Input: part model. Units: mm. Frame: model coordinates. A direction names the side the tool comes from. Coordinates: 2 decimals unless noted, no trailing zeros. Order: outer loops, then holes, each group sorted by start corner. A loop starts at its lowest first (then second) coordinate and runs counter-clockwise, first axis right, second up. Notation, with made-up numbers: (66, 3) - (122, 3) arc R32 cw to (122, 36) - close; hole circle Ø3 at (65, 4). An arc over 180 degrees is marked (long way). One line per question, with ' | ' between items. Start each with the question number.
Autodesk Fusion 360 part; units mm, degrees
sketch "Skizze1" plane through (0, 0, 0) normal (0, 1, 0) x (1, 0, 0)
  line L0 (25, 16) -> (-25, 16)
  line L1 (-25, 16) -> (-25, -16)
  line L2 (-25, -16) -> (25, -16)
  line L3 (25, -16) -> (25, 16)
  line L4 (25, 16) -> (-25, -16) construction
  line L5 (-25, 16) -> (25, -16) construction
  dimension "d1" = 50
  dimension "d2" = 32
extrude "Extrusion1" add sketch "Skizze1" along normal blind 1
sketch "Skizze2" plane through (0, 1, 0) normal (0, 1, 0) x (-1, 0, 0)
  line L0 (-25, 16) -> (-25, -16)
  line L1 (-25, -16) -> (25, -16)
  line L2 (25, -16) -> (25, 16)
  line L3 (25, 16) -> (-25, 16)
  circle A0 centre (0, 0) radius 4.9
  line L4 (0, 0) -> (0, -16) construction
  line L5 (0, 0) -> (-14.6371, -14.6371) construction
  line L6 (0, 0) -> (-14.6371, 14.6371) construction
  arc A1 (-7.0711, 7.0711) -> (-9.051, 9.051) centre (-8.061, 8.061) ccw
  arc A2 (-12.6572, 12.6572) -> (-14.6371, 14.6371) centre (-13.6472, 13.6472) ccw
  arc A3 (-9.051, 9.051) -> (-9.051, -9.051) centre (0, 0) ccw
  arc A4 (-7.0711, 7.0711) -> (-7.0711, -7.0711) centre (0, 0) ccw
  arc A5 (-14.6371, -14.6371) -> (-12.6572, -12.6572) centre (-13.6472, -13.6472) ccw
  arc A6 (-9.051, -9.051) -> (-7.0711, -7.0711) centre (-8.061, -8.061) ccw
  arc A7 (-12.6572, 12.6572) -> (-12.6572, -12.6572) centre (0, 0) ccw
  arc A8 (-14.6371, 14.6371) -> (-14.6371, -14.6371) centre (0, 0) ccw
  arc A9 (12.6572, -12.6572) -> (12.6572, 12.6572) centre (0, 0) ccw
  arc A10 (14.6371, -14.6371) -> (14.6371, 14.6371) centre (0, 0) ccw
  line L7 (25, 16) -> (25, -16)
  line L8 (0, 0) -> (14.6371, 14.6371) construction
  line L9 (25, -16) -> (-25, -16)
  arc A11 (9.051, -9.051) -> (9.051, 9.051) centre (0, 0) ccw
  arc A12 (12.6572, -12.6572) -> (14.6371, -14.6371) centre (13.6472, -13.6472) ccw
  arc A13 (7.0711, -7.0711) -> (7.0711, 7.0711) centre (0, 0) ccw
  line L10 (0, 0) -> (14.6371, -14.6371) construction
  arc A14 (9.051, 9.051) -> (7.0711, 7.0711) centre (8.061, 8.061) ccw
  line L11 (-25, 16) -> (25, 16)
  arc A15 (7.0711, -7.0711) -> (9.051, -9.051) centre (8.061, -8.061) ccw
  arc A16 (14.6371, 14.6371) -> (12.6572, 12.6572) centre (13.6472, 13.6472) ccw
  dimension "d6" = 9.8
  dimension "d7" = 2.8
  dimension "d8" = 5.1
  dimension "d9" = 5.1
  dimension "d10" = 2.8
  dimension "d11" = 45
extrude "Extrusion2" add sketch "Skizze2" along normal blind 1 contours A0 | A1 A3 A4 A6 | A2 A5 A7 A8 | A9 A10 A12 A16 | A11 A13 A14 A15
equation "d9 = d8"
equation "d10 = d7"
(1) Section A-A (y = 1.35). Output: boundary loops of the cut face in (x, z), then the cut area to 3 significant figures.
(2) Material intervals for line 1 along X through (y, z) = (1.45, -5); line 2 along X through (y, z) = (1.95, 2.5); line 3 along X through (y, z) = (1.15, -2), sorted ascending. Write a range as from..to.
(3) Draft query along Z for faces 3 (the face through (12.68, 1.49, 14.66)), 4 (the face through (-12.64, 1.49, 14.62)), 5 (the face through (0, 2, 0)), 6 (the face through (-0.3, 0.5, 16)). Return one class per face: +Z half, -Z half, draft (parallel to the pull), parting line (faces both ways), or undercut.
(4) Reachability of faces 1 (the face through (7.05, 1.49, -9.03)), 2 (the face through (-10.4, 2, 0.1)) from +Z, -Z, +X, -X, +Y, -Y: full face, straight path, thin tool, end or side. Return the list, or none.
(5) Section C-C (z = 0). Output: boundary loops of the cut face in (x, y).
(6) Section D-D (x = -20). Output: boundary loops of the cut face in (y, z).
(7) Section B-B (x = 0). Output: boundary loops of the cut face in (y, z), then the cut area to 3 significant figures.
Worked answers:
1) outline: (-14.64, -14.64) arc R1.4 ccw to (-12.66, -12.66) arc R17.9 cw to (-12.66, 12.66) arc R1.4 ccw to (-14.64, 14.64) arc R20.7 ccw to start; (-9.05, -9.05) arc R1.4 ccw to (-7.07, -7.07) arc R10 cw to (-7.07, 7.07) arc R1.4 ccw to (-9.05, 9.05) arc R12.8 ccw to start; circle Ø9.8 at (0, 0); (7.07, -7.07) arc R1.4 ccw to (9.05, -9.05) arc R12.8 ccw to (9.05, 9.05) arc R1.4 ccw to (7.07, 7.07) arc R10 cw to start; (12.66, -12.66) arc R1.4 ccw to (14.64, -14.64) arc R20.7 ccw to (14.64, 14.64) arc R1.4 ccw to (12.66, 12.66) arc R17.9 cw to start | area: 370 mm²
2) line 1: x = -20.09..-17.19, -11.78..-8.66, 8.66..11.78, 17.19..20.09 | line 2: x = -20.55..-17.72, -12.55..-9.68, -4.21..4.21, 9.68..12.55, 17.72..20.55 | line 3: x = -20.6..-17.79, -12.64..-9.8, -4.47..4.47, 9.8..12.64, 17.79..20.6
3) face 3: undercut | face 4: undercut | face 5: draft | face 6: +Z half
4) face 1: +Y | face 2: +Z, -Z, +X, -X, +Y
5) outline: (-25, 0) - (25, 0) - (25, 1) - (20.7, 1) - (20.7, 2) - (17.9, 2) - (17.9, 1) - (12.8, 1) - (12.8, 2) - (10, 2) - (10, 1) - (4.9, 1) - (4.9, 2) - (-4.9, 2) - (-4.9, 1) - (-10, 1) - (-10, 2) - (-12.8, 2) - (-12.8, 1) - (-17.9, 1) - (-17.9, 2) - (-20.7, 2) - (-20.7, 1) - (-25, 1) - close
6) outline: (0, -16) - (1, -16) - (1, -5.34) - (2, -5.34) - (2, 5.34) - (1, 5.34) - (1, 16) - (0, 16) - close
7) outline: (0, -16) - (1, -16) - (1, -4.9) - (2, -4.9) - (2, 4.9) - (1, 4.9) - (1, 16) - (0, 16) - close | area: 41.8 mm²
